```python
from build123d import *

# Parameters (mm, degrees)
F0_R     = 6
F1_DEPTH = 20.32
F2_W     = 17.0879438519
F2_H     = 13.7446504086
F3_DEPTH = 25.4
F5_DEPTH = 11.43
F7_DEPTH = 25.4
F9_DEPTH = 25.4


# Not quite as in the source:
# - a feature names something its author has since deleted; it is built from what else it names


with BuildPart() as f1:
    # F0 (on Front) → F1 (new body)
    with BuildSketch(Plane.XZ):
        Circle(F0_R)
    extrude(amount=F1_DEPTH)

    # F2 (on face) → F3 (join)
    with BuildSketch(Plane(origin=(0, 0, 0), x_dir=(-1, 0, 0), z_dir=(0, 1, 0))):
        with Locations((0.1456169412, -0.2847756259)):
            Rectangle(F2_W, F2_H)
    extrude(amount=F3_DEPTH)

    # F4 (on face) → F5 (cut)
    with BuildSketch(Plane(origin=(0, 25.4, 0), x_dir=(-1, 0, 0), z_dir=(0, 1, 0))):
        Polygon((5.5, 5.5), (0, 5.5), (-5.5, 5.5), (-5.5, -5.5), (5.5, -5.5), align=None)
    extrude(amount=-F5_DEPTH, mode=Mode.SUBTRACT)

    # F6 (on face) → F7 (cut)
    with BuildSketch(Plane(origin=(0, 0, -7.1571008302), x_dir=(1, 0, 0), z_dir=(0, 0, -1))):
        with BuildLine():
            Line((1.5748, -25.4), (1.5748, -16.734668985))
            ThreePointArc((1.5748, -16.734668985), (0, -15.159868985), (-1.5748, -16.734668985))
            ThreePointArc((-1.5748, -16.734668985), (-1.574798986, -16.7364561088), (-1.5747959439, -16.7382432303))
            Line((-1.5747959439, -16.7382432303), (-1.5649663519, -25.4))
            Line((-1.5649663519, -25.4), (1.5748, -25.4))
        make_face()
    extrude(amount=-F7_DEPTH, mode=Mode.SUBTRACT)

    # F8 (on face) → F9 (cut)
    with BuildSketch(Plane(origin=(-8.6895888671, 0, 0), x_dir=(0, -1, 0), z_dir=(-1, 0, 0))):
        with BuildLine():
            Line((-25.4, -1.5290330871), (-18.0435866661, -1.5568010835))
            ThreePointArc((-18.0435866661, -1.5568010835), (-18.0377102216, -1.5568343561), (-18.0318336934, -1.556845447))
            ThreePointArc((-18.0318336934, -1.556845447), (-16.4749882464, 0), (-18.0318336934, 1.556845447))
            ThreePointArc((-18.0318336934, 1.556845447), (-18.0377102216, 1.5568343561), (-18.0435866661, 1.5568010835))
            Line((-18.0435866661, 1.5568010835), (-25.4, 1.5290330871))
            Line((-25.4, 1.5290330871), (-25.4, -1.5290330871))
        make_face()
    extrude(amount=-F9_DEPTH, mode=Mode.SUBTRACT)


solid = f1.part
```
Check sheet for the modelled part. Datum: model origin and axes. Units: mm. A direction names the side the tool comes from. Round coordinates to 2 decimals unless told otherwise and drop trailing zeros. Order: outer loops, then holes, each group sorted by start corner. A loop starts at its lowest first (then second) coordinate and runs counter-clockwise, first axis right, second up.
1) Scan lines: line 1 (X direction, y = 21, z = -3.25); line 2 (Z direction, x = 3.75, y = 16); line 3 (Z direction, x = 0, y = -0.5). Record each from-to range of solid material in increasing order.
2) Section check B-B (x = 0). Record the boundary of the cut face in (y, z).
3) Section check C-C (y = 20). Record the boundary of the cut face in (x, z), and give its area (3 significant figures).
4) Section check A-A (z = 0). Record the boundary of the cut face in (x, y), and give its area (3 significant figures).
5) Mould release check, pull along Z, two halves, no side actions. Record for faces 4 (the cylindrical face through (-6, -10, 0)), 5 (the flat face through (3, 20, -5.5)), 6 (the flat face through (-7, 25.4, 5)): +Z half, -Z half, draft (parallel to the pull), parting line (faces both ways), or undercut.
6) Tool access check on faces 1 (the flat face through (-5.5, 20, -3)), 2 (the flat face through (-4, 0, -5)), 3 (the flat face through (1.575, 21, -6)). Record the directions out of +Z, -Z, +X, -X, +Y, -Y that give a thin tool (end or side, any length) a straight path to the whole face; none if there is none.
Result:
1. line 1: x = -8.69 to -5.5, 5.5 to 8.4
1. line 2: z = -7.16 to -5.5, 5.5 to 6.59
1. line 3: z = -6 to 6
2. outline: (-20.32, -6) - (0, -6) - (0, -7.16) - (15.16, -7.16) - (15.16, -5.5) - (13.97, -5.5) - (13.97, 5.5) - (15.16, 5.5) - (15.16, 6.59) - (0, 6.59) - (0, 6) - (-20.32, 6) - close
3. outline: (-8.69, -7.16) - (-1.57, -7.16) - (-1.57, -5.5) - (-5.5, -5.5) - (-5.5, -1.55) - (-8.69, -1.55) - close; (-8.69, 1.55) - (-5.5, 1.55) - (-5.5, 5.5) - (-1.57, 5.5) - (-1.57, 6.59) - (-8.69, 6.59) - close; (1.57, -7.16) - (8.4, -7.16) - (8.4, -1.55) - (5.5, -1.55) - (5.5, -5.5) - (1.57, -5.5) - close; (1.57, 5.5) - (5.5, 5.5) - (5.5, 1.55) - (8.4, 1.55) - (8.4, 6.59) - (1.57, 6.59) - close
3. area: 86.4 mm2
4. outline: (-8.69, 0) - (-6, 0) - (-6, -20.32) - (6, -20.32) - (6, 0) - (8.4, 0) - (8.4, 16.47) - (5.5, 16.47) - (5.5, 13.97) - (-5.5, 13.97) - (-5.5, 16.47) - (-8.69, 16.47) - close
4. area: 498 mm2
5. face 4: parting line
5. face 5: undercut
5. face 6: draft
6. face 1: +Y
6. face 2: -Y
6. face 3: +Z, -Z, +Y
